```python
from build123d import *

# Parameters (mm, degrees)
CUT_EXTRUDE_1_DEPTH      = 169.683134901
SKETCH_4_R               = 15
CUT_EXTRUDE_2_DEPTH      = 165.033533157
PATTERN_CIRCULAR_1_COUNT = 6
CHAMFER_1_SIZE           = 1
CHAMFER_2_SIZE           = 1
FILLET_1_R               = 3
FILLET_2_R               = 3


with BuildPart() as part:
    # 草图2 → 旋转1 (revolve)
    with BuildSketch(Plane(origin=(0, 0, 0), x_dir=(0, 0, -1), z_dir=(1, 0, 0)), mode=Mode.PRIVATE) as revolve_1_sk:
        Polygon((0, 0), (0, 18.342006946), (32, 18.342006946), (32, 1.342006946), (98, 1.342006946), (98, 18.342006946), (113, 18.342006946), (113, -13.309731327), (113, -35.657993054), (98, -35.657993054), (98, -18.657993054), (32, -18.657993054), (32, -35.657993054), (0, -35.657993054), (0, -10.537464958), align=None)
    revolve(revolve_1_sk.sketch.rotate(Axis((0, -10.537464958, 0), (0, -1, 0)), 180), axis=Axis((0, -10.537464958, 0), (0, -1, 0)))

    # 草图3 → 切除-拉伸1 (cut, through all)
    with BuildSketch(Plane(origin=(0, 18.342006946, 0), x_dir=(1, 0, 0), z_dir=(0, 1, 0))):
        with BuildLine():
            Line((-5, 18.33030278), (-5, 22.3))
            Line((-5, 22.3), (5, 22.3))
            Line((5, 22.3), (5, 18.33030278))
            ThreePointArc((5, 18.33030278), (0, -19), (-5, 18.33030278))
        make_face()
    extrude(amount=-CUT_EXTRUDE_1_DEPTH, mode=Mode.SUBTRACT)

    # 草图4 → 切除-拉伸2 (cut, through all)
    with BuildSketch(Plane(origin=(0, 1.342006946, 0), x_dir=(1, 0, 0), z_dir=(0, 1, 0))):
        with Locations(Location((0, 65, 0), (0, 0, 270))):
            Circle(SKETCH_4_R)
    cut_extrude_2 = extrude(amount=-CUT_EXTRUDE_2_DEPTH, mode=Mode.SUBTRACT)

    # 阵列(圆周)1: 切除-拉伸2 ×6 about axis
    pattern_circular_1_axis = Axis((0, 0, 0), (0, 1, 0))
    for i in range(1, PATTERN_CIRCULAR_1_COUNT):
        add(cut_extrude_2.rotate(pattern_circular_1_axis, i * 360 / PATTERN_CIRCULAR_1_COUNT), mode=Mode.SUBTRACT)

    # 倒角1
    chamfer_1_edges = [part.edges().sort_by_distance(p)[0] for p in [
        (0, -35.657993054, -113),
        (0, 18.342006946, -113),
    ]]
    chamfer(chamfer_1_edges, length=CHAMFER_1_SIZE)

    # 倒角2
    chamfer_2_edges = [part.edges().sort_by_distance(p)[0] for p in [
        (0, -35.657993054, -32),
        (0, -18.657993054, -98),
        (0, -35.657993054, -98),
        (0, 18.342006946, -98),
        (0, 1.342006946, -98),
        (0, 18.342006946, -32),
        (0, -35.657993054, 19),
        (0, 18.342006946, 19),
    ]]
    chamfer(chamfer_2_edges, length=CHAMFER_2_SIZE)

    # 圆角1
    fillet_1_edges = [part.edges().sort_by_distance(p)[0] for p in [
        (0, 1.342006946, -32),
        (0, 17.342006946, -32),
    ]]
    fillet(fillet_1_edges, radius=FILLET_1_R)

    # 圆角2
    fillet_2_edges = [part.edges().sort_by_distance(p)[0] for p in [
        (0, -18.657993054, -32),
        (0, -34.657993054, -32),
    ]]
    fillet(fillet_2_edges, radius=FILLET_2_R)


solid = part.part
```
Source: CAD feature listing. Evaluate the final solid. Frame: model axes, mm. A direction names the side the tool comes from. Give positions to 0.01 mm unless a question says otherwise; leave off trailing zeros. Order: outer loops, then holes, each group sorted by start corner. A loop starts at its lowest first (then second) coordinate and runs counter-clockwise, first axis right, second up.
(1) Section query A-A (y = 10). Return the cut outline in (x, z).
(2) Section query B-B (x = 0). State how many separate pieces and enclosed holes the cut face has, plus the area to 3 significant figures.
(3) Section query C-C (y = -4). Return the cut outline in (x, z).
(4) Access query for faces 5 (the face through (-1, 1.342, -42)), 6 (the face through (31.24, -27.62, -6.94)), 7 (the face through (0, -8, -22.3)). Directions: +Z, -Z, +X, -X, +Y, -Y. A direction counts if a zero-diameter tool reaches every point of the face in a straight line with its end or side. Return the directions, or none.
(5) Pull-direction query (Z, two-part tool) for faces 1 (the face through (99, 18.342, -8)), 2 (the face through (0.77, 17.5, 19.14)), 3 (the face through (41.42, -8.52, -30.55)), 4 (the face through (-33.942, -8.294, 107.782)); classes: +Z half, -Z half, draft (parallel to the pull), parting line (faces both ways), or undercut.
(6) Material intervals for line 1 along X through (y, z) = (-19.5, -26); line 2 along Z through (x, y) = (-61.5, -17.5); line 3 along Z through (x, y) = (-25, -24.5), sorted ascending.
(7) Contact query for flat-ended pins moving along their axis: P1, Ø3, axis at x = -13, y = -21.5, coming from the +Z side; P2, Ø12, axis at y = -12, z = -19, coming from the +X side; P3, Ø2, axis at y = 8.5, z = 6.5, coming from the +X side. Output: stop coordinate, or through.
Outcome:
1. outline: circle Ø226 at (0, 0); circle Ø64 at (0, 0); hole circle Ø196 at (0, 0); hole (-5, -22.3) - (5, -22.3) - (5, -18.33) arc R19 ccw (long way) to (-5, -18.33) - close
2. separate pieces: 4
2. enclosed holes: 0
2. area: 4,290 mm2
3. outline: circle Ø226 at (0, 0); hole circle Ø30 at (-56.29, -32.5); hole circle Ø30 at (-56.29, 32.5); hole circle Ø30 at (0, -65); hole circle Ø30 at (0, 65); hole (-5, -22.3) - (5, -22.3) - (5, -18.33) arc R19 ccw (long way) to (-5, -18.33) - close; hole circle Ø30 at (56.29, -32.5); hole circle Ø30 at (56.29, 32.5)
4. face 5: +Y
4. face 6: -Y
4. face 7: +Y, -Y
5. face 1: draft
5. face 2: undercut
5. face 3: undercut
5. face 4: parting line
6. line 1: x = -109.97 to -94.32, -20.19 to 20.19, 94.32 to 109.97
6. line 2: z = -94.8 to -46.57, -18.43 to 18.43, 46.57 to 94.8
6. line 3: z = -110.2 to -94.76, -19.97 to 19.97, 94.76 to 110.2
7. P1: stops at z = 112.41
7. P2: stops at x = 112.25
7. P3: stops at x = 112.87
